from build123d import *

# Parameters (mm, degrees)
SKETCH_1_W      = 10
SKETCH_1_H      = 2.85
EXTRUDE_1_DEPTH = 3
FILLET_1_R      = 1
FILLET_2_R      = 0.5


with BuildPart() as part:
    # Эскиз1 → Бобышка-Вытянуть1 (new body)
    with BuildSketch(Plane(origin=(0, 0, 0), x_dir=(0, 0, -1), z_dir=(1, 0, 0))):
        Polygon((-10.5, -40), (10.5, -40), (10.5, 40), (-10.5, 40), (-10.5, -26), (-13.35, -26), (-13.35, -29), (-10.5, -29), align=None)
        with Locations((0, 5.5)):
            Rectangle(SKETCH_1_W, SKETCH_1_H, mode=Mode.SUBTRACT)
        with Locations((0, -35.5)):
            Rectangle(SKETCH_1_W, SKETCH_1_H, mode=Mode.SUBTRACT)
        with Locations((0, 35.5)):
            Rectangle(SKETCH_1_W, SKETCH_1_H, mode=Mode.SUBTRACT)
    extrude(amount=EXTRUDE_1_DEPTH)

    # Скругление1
    fillet_1_edges = [part.edges().sort_by_distance(p)[0] for p in [
        (1.5, -40, -10.5),
        (1.5, -40, 10.5),
        (1.5, 40, 10.5),
        (1.5, 40, -10.5),
    ]]
    fillet(fillet_1_edges, radius=FILLET_1_R)

    # Скругление2
    fillet_2_edges = [part.edges().sort_by_distance(p)[0] for p in [
        (1.5, -29, 13.35),
        (1.5, -26, 13.35),
    ]]
    fillet(fillet_2_edges, radius=FILLET_2_R)


solid = part.part
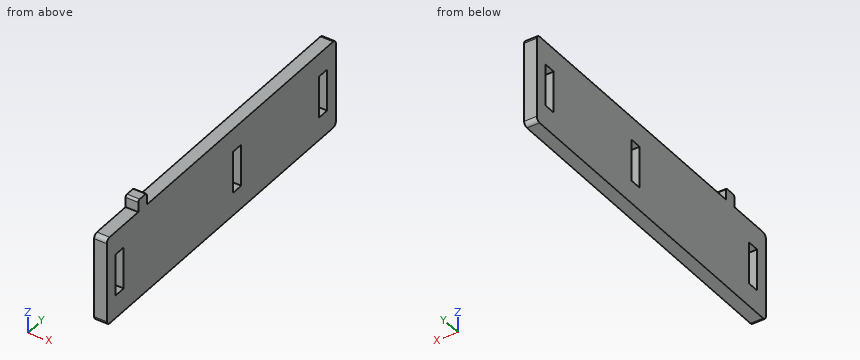
Input: part model. Units: mm. Frame: model coordinates. Round coordinates to 2 decimals unless told otherwise and drop trailing zeros. Loops run counter-clockwise (first coordinate to the right, second up) from the corner with the lowest first, then second, coordinate; pieces in that order, holes last. Notation, with made-up numbers: M 11,-10.75 L 39,-10.75 A26 ccw 39,10.25 Z; hole C -32,57.5 d10. An arc over 180 degrees is marked long. Answer as CSV lines item,"result". Start each with the question number.
(1) Section C-C, the plane y = -22. Output: boundary loops of the cut face in (x, z), plus the area to 3 significant figures.
(2) Section A-A, the plane z = 2. Output: boundary loops of the cut face in (x, y) (3 decimals).
(3) Line query: line 1 (Y direction, x = 1.3, z = 4.75) (3 decimals); line 2 (Z direction, x = 2.5, y = 35); line 3 (Z direction, x = 2.1, y = 30). Output: solid intervals per line, ascending. Write a range as [from, to].
(4) First-contact query: pin 1 (0.9 mm diameter, centred on x = 1, y = -35.5, fed in from +Z); pin 2 (1.2 mm diameter, centred on x = 1.5, z = 12, fed in from -Y); pin 3 (1.5 mm diameter, centred on x = 1.5, z = 10.5, fed in from +Y). Flat tips, straight axial feed; report the tip coordinate or a pass-through.
(5) Section B-B, the plane x = 2.5. Output: boundary loops of the cut face in (y, z) (3 decimals).
Values found:
1,outline,"M 0,-10.5 L 3,-10.5 L 3,10.5 L 0,10.5 Z"
1,area,"63.0 mm²"
2,outline,"M 0,-40 L 3,-40 L 3,-36.925 L 0,-36.925 Z; M 0,-34.075 L 3,-34.075 L 3,4.075 L 0,4.075 Z; M 0,6.925 L 3,6.925 L 3,34.075 L 0,34.075 Z; M 0,36.925 L 3,36.925 L 3,40 L 0,40 Z"
3,line 1,"y = [-40, -36.925], [-34.075, 4.075], [6.925, 34.075], [36.925, 40]"
3,line 2,"z = [-10.5, -5], [5, 10.5]"
3,line 3,"z = [-10.5, 10.5]"
4,pin 1,"stops at z = 10.5"
4,pin 2,"stops at y = -29"
4,pin 3,"stops at y = 39.97"
5,outline,"M -40,-9.5 A1 ccw -39,-10.5 L 39,-10.5 A1 ccw 40,-9.5 L 40,9.5 A1 ccw 39,10.5 L -26,10.5 L -26,12.85 A0.5 ccw -26.5,13.35 L -28.5,13.35 A0.5 ccw -29,12.85 L -29,10.5 L -39,10.5 A1 ccw -40,9.5 Z; hole M -36.925,-5 L -34.075,-5 L -34.075,5 L -36.925,5 Z; hole M 4.075,-5 L 6.925,-5 L 6.925,5 L 4.075,5 Z; hole M 34.075,-5 L 36.925,-5 L 36.925,5 L 34.075,5 Z"
